Check sheet for the drawn part. Datum: minimum x, y, z corner. Units: mm. A direction names the side the tool comes from. Give positions to 0.01 mm unless a question says otherwise; leave off trailing zeros. Loops run counter-clockwise (first coordinate to the right, second up) from the corner with the lowest first, then second, coordinate; pieces in that order, holes last.
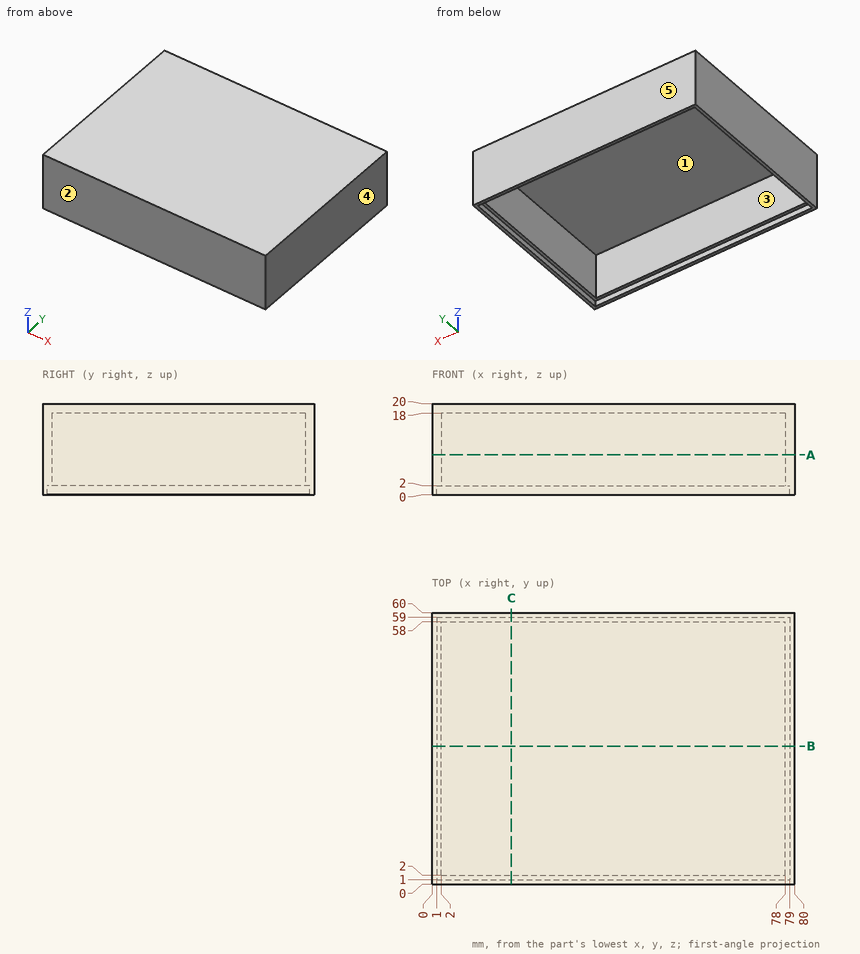
1) Sectioned sample at A-A on z = 8.75. Enter the section's corners in (x, y).
2) Scan lines: line 1 along Y through (x, z) = (76, 14); line 2 along X through (y, z) = (4, 12); line 3 along X through (y, z) = (21.5, 1.25). Record each from-to range of solid material in increasing order.
3) Tool access check on the marked faces 1 and 2. Record the directions out of +Z, -Z, +X, -X, +Y, -Y that give a thin tool (end or side, any length) a straight path to the whole face; none if there is none.
4) Sectioned sample at C-C on x = 17.5. Enter the section's corners in (y, z).
5) Mould release check, pull along X, two halves, no side actions. Record for the marked faces 3, 4 and 5: +X half, -X half, draft (parallel to the pull), parting line (faces both ways), or undercut.
6) Sectioned sample at B-B on y = 30.5. Enter the section's corners in (x, z).
7) Depth check by flat-ended pin: P1, Ø5, axis at x = 45.5, z = 7.5, coming from the -Y side; P2, Ø17, axis at x = 37, y = 19.5, coming from the -Z side. Enter the tip coordinate at first touch or a pass-through.
Determined:
1. outline: (0, 0) - (80, 0) - (80, 60) - (0, 60) - close; hole (2, 2) - (78, 2) - (78, 58) - (2, 58) - close
2. line 1: y = 0 to 2, 58 to 60
2. line 2: x = 0 to 2, 78 to 80
2. line 3: x = 0 to 1, 79 to 80
3. face 1: -Z
3. face 2: +Z, -Z, +X, -X, -Y
4. outline: (0, 0) - (1, 0) - (1, 2) - (2, 2) - (2, 18) - (58, 18) - (58, 2) - (59, 2) - (59, 0) - (60, 0) - (60, 20) - (0, 20) - close
5. face 3: undercut
5. face 4: +X half
5. face 5: draft
6. outline: (0, 0) - (1, 0) - (1, 2) - (2, 2) - (2, 18) - (78, 18) - (78, 2) - (79, 2) - (79, 0) - (80, 0) - (80, 20) - (0, 20) - close
7. P1: stops at y = 0
7. P2: stops at z = 18
